Geometry: final body of the model. Coordinates: model frame, mm. Face numbers are marked on the shaded views. A direction names the side the tool comes from. Give positions to 0.01 mm unless a question says otherwise; leave off trailing zeros. Write each loop counter-clockwise with the first axis right and the second up, starting at its lowest first coordinate (ties: lowest second). Pieces come first, ordered by that corner, then holes. Notation, with made-up numbers: (5, 54.25) -> (48, 54.25) arc R14 cw to (48, 81.25) -> close; hole circle Ø3 at (16.25, 36). An arc over 180 degrees is marked (long way). Answer as a JSON object with one key per item and string values. Group by question number.
(1) Draft query along Z for the marked faces 4, 5 and 6. Return one class per face: +Z half, -Z half, draft (parallel to the pull), parting line (faces both ways), or undercut.
(2) Section query C-C on x = 23. Output: boundary loops of the cut face in (y, z).
(3) Set-up query: the marked faces 1, 2 and 3. Return all of +Z, -Z, +X, -X, +Y, -Y with unobstructed straight access to the full face (end or side cutting, diameter ignored); none if empty.
(4) Section query A-A on y = -18. Output: boundary loops of the cut face in (x, z).
(5) Section query D-D on x = -22.5. Output: boundary loops of the cut face in (y, z).
(6) Contact query for flat-ended pins moving along their axis: pin 1 Ø0.6 at (y, z) = (35.5, 14) entering from -X; pin 2 Ø5 at (x, z) = (-21, 3) entering from -Y; pin 3 Ø10 at (x, z) = (-6.5, 10) entering from -Y. Output: stop coordinate, or through.
(7) Material intervals for probe 1 along X at (y, z) = (-34, 7.25); probe 2 along Y at (x, z) = (1, 6.25); probe 3 along Z at (x, y) = (-4, -3.5), sorted ascending.
(8) Section query B-B on y = -2.5. Output: boundary loops of the cut face in (x, z), plus the area to 3 significant figures.
from build123d import *

# Parameters (mm, degrees)
F1_DEPTH    = 25
F3_R        = 2.54
F4_W        = 50
F4_H        = 30
F5_DEPTH    = 20
F2_W        = 12.7
F2_H        = 25
F6_DEPTH    = 25
F7_T        = -2
F8_T1_DEPTH = 75.655609521
F10_W       = 5
F10_H       = 15
F11_DEPTH   = 10
F12_W       = 7.3
F12_H       = 11.5
F13_DEPTH   = 25.4
F16_R       = 4.25
F18_W       = 5
F18_H       = 3
F19_DEPTH   = 3


# Not quite as in the source:
# - a fillet or chamfer that OpenCascade refuses, or shapes differently, is made with other operations: its cross-section is extruded or revolved along the edge and cut away or added
# - a feature names something its author has since deleted; it is built from what else it names


with BuildPart() as f1:
    # F0 (on Top) → F1 (new body)
    with BuildSketch(Plane.XY):
        with BuildLine():
            Line((30, -36.5978047605), (30, 36.5978047605))
            Line((30, 36.5978047605), (-30, 36.5978047605))
            Line((-30, 36.5978047605), (-30, -36.5978047605))
            ThreePointArc((-30, -36.5978047605), (0, -46.4021952395), (30, -36.5978047605))
        make_face()
    extrude(amount=F1_DEPTH)

    # F3
    f3_edges = [f1.edges().sort_by_distance(p)[0] for p in [
        (-30, 36.597805, 12.5),
        (30, 36.597805, 12.5),
    ]]
    fillet(f3_edges, radius=F3_R)

    # F4 (on face) → F5 (cut)
    with BuildSketch(Plane.XY):
        with Locations((0, -31.4021952395)):
            Rectangle(F4_W, F4_H)
    extrude(amount=F5_DEPTH, mode=Mode.SUBTRACT)

    # F2 (on Top) → F6 (cut, through all)
    with BuildSketch(Plane.XY):
        with Locations((0, -33.9021952395)):
            Rectangle(F2_W, F2_H)
    extrude(amount=F6_DEPTH, mode=Mode.SUBTRACT)

    # F7 (hollow: no face is removed)
    offset(amount=F7_T, kind=Kind.INTERSECTION, mode=Mode.SUBTRACT)

    # F8: fillet of radius 1 on 4 edges, made by hand

    # F8_s2 → F8_t1 (cut)
    with BuildSketch(Plane.XZ.offset(-36.5578047605)):
        with BuildLine():
            ThreePointArc((29, 0), (29.7071067812, 0.2928932188), (30, 1))
            Line((30, 1), (30, 0))
            Line((30, 0), (29, 0))
        make_face()
        with BuildLine():
            ThreePointArc((29, 25), (29.7071067812, 24.7071067812), (30, 24))
            Line((30, 24), (30, 25))
            Line((30, 25), (29, 25))
        make_face()
        with BuildLine():
            ThreePointArc((-29, 25), (-29.7071067812, 24.7071067812), (-30, 24))
            Line((-30, 24), (-30, 25))
            Line((-30, 25), (-29, 25))
        make_face()
        with BuildLine():
            ThreePointArc((-29, 0), (-29.7071067812, 0.2928932188), (-30, 1))
            Line((-30, 1), (-30, 0))
            Line((-30, 0), (-29, 0))
        make_face()
    extrude(amount=F8_T1_DEPTH, mode=Mode.SUBTRACT)

    # F10 (on face) → F11 (cut)
    with BuildSketch(Plane(origin=(0, 36.5978047605, 0), x_dir=(-1, 0, 0), z_dir=(0, 1, 0))):
        with Locations((-15.5, 12.5)):
            Rectangle(F10_W, F10_H)
        with Locations((15.5, 12.5)):
            Rectangle(F10_W, F10_H)
        with Locations((-5.5, 12.5)):
            Rectangle(F10_W, F10_H)
        with Locations((5.5, 12.5)):
            Rectangle(F10_W, F10_H)
    extrude(amount=-F11_DEPTH, mode=Mode.SUBTRACT)

    # F12 (on face) → F13 (cut)
    with BuildSketch(Plane(origin=(0, 36.5978047605, 0), x_dir=(-1, 0, 0), z_dir=(0, 1, 0))):
        with Locations((23.35, 12.5)):
            Rectangle(F12_W, F12_H)
    extrude(amount=-F13_DEPTH, mode=Mode.SUBTRACT)

    # F17: sweep along a path in F15
    with BuildLine(Plane.XY.offset(12)) as f17_path:
        Line((-13, -16.4021952395), (-13, -28.9021952395))
        ThreePointArc((-13, -28.9021952395), (0, -41.9021952395), (13, -28.9021952395))
        Line((13, -28.9021952395), (13, -16.4021952395))
    # F16 (on face) → F17 (sweep)
    with BuildSketch(Plane.XZ.offset(16.4021952395)):
        with Locations((-13.0000123754, 11.9999870658)):
            Circle(F16_R)
    sweep(path=f17_path.line)

    # F18 (on face) → F19 (cut)
    with BuildSketch(Plane.XY.offset(25)):
        with Locations((27.5, 25.0978047605)):
            Rectangle(F18_W, F18_H)
        with Locations((27.5, 19.0978047605)):
            Rectangle(F18_W, F18_H)
    extrude(amount=-F19_DEPTH, mode=Mode.SUBTRACT)


solid = f1.part
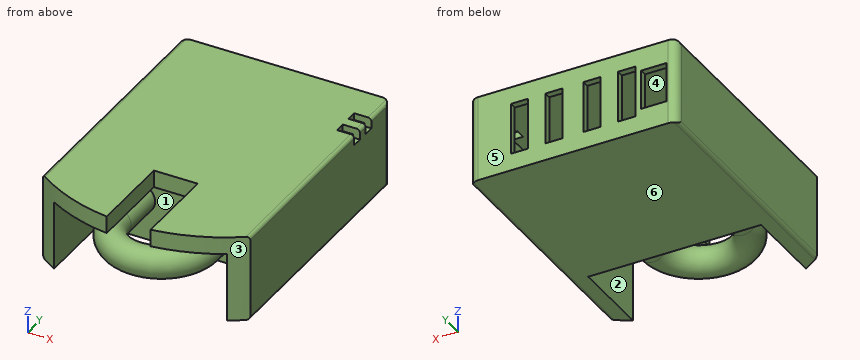
Answer list:
{
 "1": {"face 4": "undercut", "face 5": "draft", "face 6": "-Z half"},
 "2": {"outline": "(-40.9, 20) -> (-16.4, 20) -> (-16.4, 0) -> (36.6, 0) -> (36.6, 25) -> (-40.9, 25) -> close; hole (-38.64, 22) -> (-14.4, 22) -> (-14.4, 2) -> (34.6, 2) -> (34.6, 23) -> (-38.64, 23) -> close"},
 "3": {"face 1": "none", "face 2": "-Z, -Y", "face 3": "+Z, -Z, +X, -Y"},
 "4": {"outline": "(-30, 1) arc R1 ccw to (-29, 0) -> (-25, 0) -> (-25, 20) -> (25, 20) -> (25, 0) -> (29, 0) arc R1 ccw to (30, 1) -> (30, 24) arc R1 ccw to (29, 25) -> (-29, 25) arc R1 ccw to (-30, 24) -> close; circle Ø8.5 at (-13, 12); circle Ø8.5 at (13, 12); hole (-28, 2) -> (-27, 2) -> (-27, 22) -> (27, 22) -> (27, 2) -> (28, 2) -> (28, 23) -> (-28, 23) -> close"},
 "5": {"outline": "(-41.15, 20) -> (-16.4, 20) -> (-16.4, 0) -> (36.6, 0) -> (36.6, 6.75) -> (34.6, 6.75) -> (34.6, 2) -> (-14.4, 2) -> (-14.4, 22) -> (-38.91, 22) -> (-38.91, 23) -> (34.6, 23) -> (34.6, 18.25) -> (36.6, 18.25) -> (36.6, 25) -> (-41.15, 25) -> close"},
 "6": {"pin 1": "x = -29.73", "pin 2": "y = -16.4", "pin 3": "y = -46.05"},
 "7": {"probe 1": "-30 to -28, -27 to -25, 25 to 27, 28 to 30", "probe 2": "-16.4 to -14.4, 34.6 to 36.6", "probe 3": "0 to 2, 23 to 25"},
 "8": {"outline": "(-30, 1) arc R1 ccw to (-29, 0) -> (29, 0) arc R1 ccw to (30, 1) -> (30, 24) arc R1 ccw to (29, 25) -> (-29, 25) arc R1 ccw to (-30, 24) -> close; hole (-28, 2) -> (28, 2) -> (28, 23) -> (-28, 23) -> close", "area": "323 mm2"}
}
